Here's how the part is built. I have some questions about the finished solid (model axes, mm). A direction names the side the tool comes from. Coordinates: 2 decimals unless noted, no trailing zeros. Write each loop counter-clockwise with the first axis right and the second up, starting at its lowest first coordinate (ties: lowest second). Pieces come first, ordered by that corner, then holes. Notation, with made-up numbers: M 65,-1.5 L 71,-1.5 A24 ccw 71,18.5 Z; hole C 7.5,23.5 d7. An arc over 180 degrees is marked long. Use a Markdown table: item, result.
```python
from build123d import *

# Parameters (mm, degrees)
F0_W     = 150
F0_H     = 150
F1_DEPTH = 5
F2_R     = 18.25
F3_DEPTH = 2.5
F4_R     = 11
F5_DEPTH = 5
F6_R     = 2
F7_DEPTH = 5.001


with BuildPart() as f1:
    # F0 (on Top) → F1 (new body)
    with BuildSketch(Plane.XY):
        Rectangle(F0_W, F0_H)
    extrude(amount=-F1_DEPTH)

    # F2 (on face) → F3 (join)
    with BuildSketch(Plane.XY):
        Circle(F2_R)
    extrude(amount=F3_DEPTH)

    # F4 (on face) → F5 (join)
    with BuildSketch(Plane.XY):
        with Locations((-39.25, 0)):
            Circle(F4_R)
        with BuildLine():
            Line((37.714466, 12.535534), (28.714466, 3.535534))
            ThreePointArc((28.714466, 3.535534), (27.25, 0), (28.714466, -3.535534))
            Line((28.714466, -3.535534), (37.714466, -12.535534))
            ThreePointArc((37.714466, -12.535534), (41.25, -14), (44.785534, -12.535534))
            Line((44.785534, -12.535534), (53.785534, -3.535534))
            ThreePointArc((53.785534, -3.535534), (55.25, 0), (53.785534, 3.535534))
            Line((53.785534, 3.535534), (44.785534, 12.535534))
            ThreePointArc((44.785534, 12.535534), (41.25, 14), (37.714466, 12.535534))
        make_face()
    extrude(amount=F5_DEPTH)

    # F6 (on face) → F7 (cut, through all)
    with BuildSketch(Plane.XY):
        with Locations((0, 28.5)):
            Circle(F6_R)
        with Locations((-24.681724, 14.25)):
            Circle(F6_R)
        with Locations((-24.681724, -14.25)):
            Circle(F6_R)
        with Locations((0, -28.5)):
            Circle(F6_R)
        with Locations((24.681724, -14.25)):
            Circle(F6_R)
        with Locations((24.681724, 14.25)):
            Circle(F6_R)
    extrude(amount=-F7_DEPTH, mode=Mode.SUBTRACT)


solid = f1.part
```
1. Suppose I cut it at C-C on x = -39.25. Write out the boundary of the cut face in (y, z), and give its area (3 significant figures).
Answers follow:
| item | result |
|---|---|
| outline | M -75,-5 L 75,-5 L 75,0 L 11,0 L 11,5 L -11,5 L -11,0 L -75,0 Z |
| area | 860 mm2 |
2. Suppose I cut it at A-A on y = -28.5. Write out the boundary of the cut face in (x, z), and give its area (3 significant figures).
Answers follow:
| item | result |
|---|---|
| outline | M -75,-5 L -2,-5 L -2,0 L -75,0 Z; M 2,-5 L 75,-5 L 75,0 L 2,0 Z |
| area | 730 mm2 |
3. Will these pins go through, and if not, where does the flat tip stop? pin 1 Ø2.5 at (x, y) = (24.68, -14.25) entering from -Z; pin 2 Ø6 at (x, z) = (-9.5, 4) entering from -Y; pin 3 Ø5 at (x, y) = (-24.68, 14.25) entering from +Z.
Answers follow:
| item | result |
|---|---|
| pin 1 | passes through |
| pin 2 | stops at y = -16.89 |
| pin 3 | stops at z = 0 |
4. I need wall thicknesses on probe 1 along Y at (x, z) = (0, -1.85); probe 2 along Z at (x, y) = (32, 49.5); probe 3 along X at (y, z) = (-12.5, -3). Which ranges of each line are inside material? Lowest first, please.
Answers follow:
| item | result |
|---|---|
| probe 1 | y = -75 to -30.5, -26.5 to 26.5, 30.5 to 75 |
| probe 2 | z = -5 to 0 |
| probe 3 | x = -75 to -25.65, -23.71 to 23.71, 25.65 to 75 |
5. Which directions (+Z, -Z, +X, -X, +Y, -Y) give clear straight access to the entire face, cutting with the end or side of a thin tool? Please do faces 1 (the face through (41.2, -14, 2.5)), 2 (the face through (41.3, 14, 2.5)), 3 (the face through (-18, 18, 0)), 4 (the face through (55.25, -0.05, 2.46)), 5 (the face through (0, 0, 2.5)).
Answers follow:
| item | result |
|---|---|
| face 1 | +Z, -Y |
| face 2 | +Z, +Y |
| face 3 | +Z |
| face 4 | +Z, +X |
| face 5 | +Z, +Y, -Y |
6. Suppose I cut it at D-D on y = 0. Write out the boundary of the cut face in (x, z), and give its area (3 significant figures).
Answers follow:
| item | result |
|---|---|
| outline | M -75,-5 L 75,-5 L 75,0 L 55.25,0 L 55.25,5 L 27.25,5 L 27.25,0 L 18.25,0 L 18.25,2.5 L -18.25,2.5 L -18.25,0 L -28.25,0 L -28.25,5 L -50.25,5 L -50.25,0 L -75,0 Z |
| area | 1,090 mm2 |
7. Suppose I cut it at B-B on x = 0. Write out the boundary of the cut face in (y, z).
Answers follow:
| item | result |
|---|---|
| outline | M -75,-5 L -30.5,-5 L -30.5,0 L -75,0 Z; M -26.5,-5 L 26.5,-5 L 26.5,0 L 18.25,0 L 18.25,2.5 L -18.25,2.5 L -18.25,0 L -26.5,0 Z; M 30.5,-5 L 75,-5 L 75,0 L 30.5,0 Z |
8. We'd pull the mould along X, two halves only. Please class faces 6 (the face through (33.15, -7.97, 2.46)), 7 (the face through (49.22, -8.1, 2.46)), 8 (the face through (27.25, 0.05, 2.46)), 9 (the face through (41, 0, 5)): +X half, -X half, draft (parallel to the pull), parting line (faces both ways), or undercut.
Answers follow:
| item | result |
|---|---|
| face 6 | undercut |
| face 7 | +X half |
| face 8 | undercut |
| face 9 | draft |
